Part print with two shaded views. Sizes in mm from the minimum x, y, z corner. Round coordinates to 2 decimals unless told otherwise and drop trailing zeros. Loops run counter-clockwise (first coordinate to the right, second up) from the corner with the lowest first, then second, coordinate; pieces in that order, holes last. Notation, with made-up numbers: (78.5, 66.5) - (107.5, 66.5) arc R9 cw to (107.5, 70.5) - close; hole circle Ø2 at (87.5, -32). An arc over 180 degrees is marked (long way). Use a Markdown table: item, result.
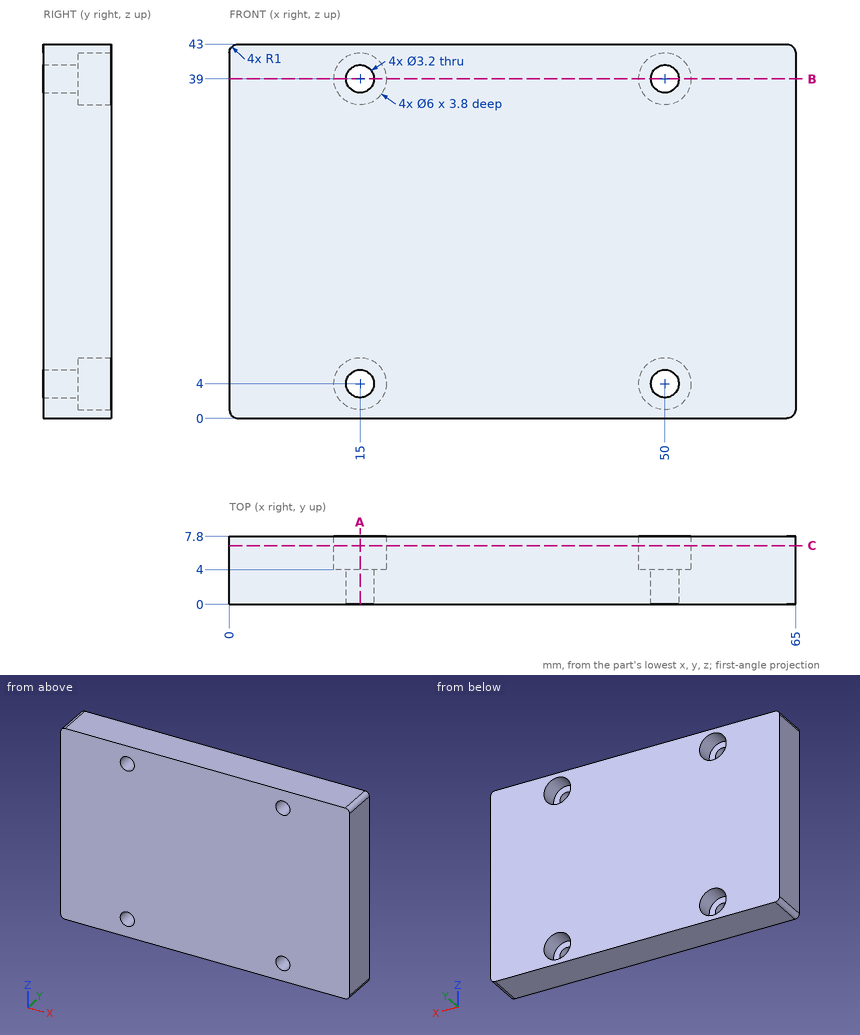
Q1. Cut at C-C, the plane y = 6.75. List the corners of the cut face in (x, z), plus the area to 3 significant figures.
Results found:
| item | result |
|---|---|
| outline | (0, 1) arc R1 ccw to (1, 0) - (64, 0) arc R1 ccw to (65, 1) - (65, 42) arc R1 ccw to (64, 43) - (1, 43) arc R1 ccw to (0, 42) - close; hole circle Ø6 at (15, 4); hole circle Ø6 at (15, 39); hole circle Ø6 at (50, 4); hole circle Ø6 at (50, 39) |
| area | 2,680 mm2 |
Q2. Drop flat-ended pins along their axis: pin 1 (1.8 mm diameter, centred on x = 50, z = 39, fed in from +Y); pin 2 (3 mm diameter, centred on x = 15.5, z = 40, fed in from +Y). Give the stop position or say it passes through.
Results found:
| item | result |
|---|---|
| pin 1 | passes through |
| pin 2 | stops at y = 4 |
Q3. Probe line 1 (X direction, y = 4.85, z = 39); line 2 (X direction, y = 0.8, z = 39); line 3 (Z direction, x = 15, y = 1.7). List the from-to ranges inside material, lowest first.
Results found:
| item | result |
|---|---|
| line 1 | x = 0 to 12, 18 to 47, 53 to 65 |
| line 2 | x = 0 to 13.4, 16.6 to 48.4, 51.6 to 65 |
| line 3 | z = 0 to 2.4, 5.6 to 37.4, 40.6 to 43 |
Q4. Cut at A-A, the plane x = 15. List the corners of the cut face in (y, z).
Results found:
| item | result |
|---|---|
| outline | (0, 0) - (7.8, 0) - (7.8, 1) - (4, 1) - (4, 2.4) - (0, 2.4) - close; (0, 5.6) - (4, 5.6) - (4, 7) - (7.8, 7) - (7.8, 36) - (4, 36) - (4, 37.4) - (0, 37.4) - close; (0, 40.6) - (4, 40.6) - (4, 42) - (7.8, 42) - (7.8, 43) - (0, 43) - close |
Q5. Cut at B-B, the plane z = 39. List the corners of the cut face in (x, y), plus the area to 3 significant figures.
Results found:
| item | result |
|---|---|
| outline | (0, 0) - (13.4, 0) - (13.4, 4) - (12, 4) - (12, 7.8) - (0, 7.8) - close; (16.6, 0) - (48.4, 0) - (48.4, 4) - (47, 4) - (47, 7.8) - (18, 7.8) - (18, 4) - (16.6, 4) - close; (51.6, 0) - (65, 0) - (65, 7.8) - (53, 7.8) - (53, 4) - (51.6, 4) - close |
| area | 436 mm2 |
